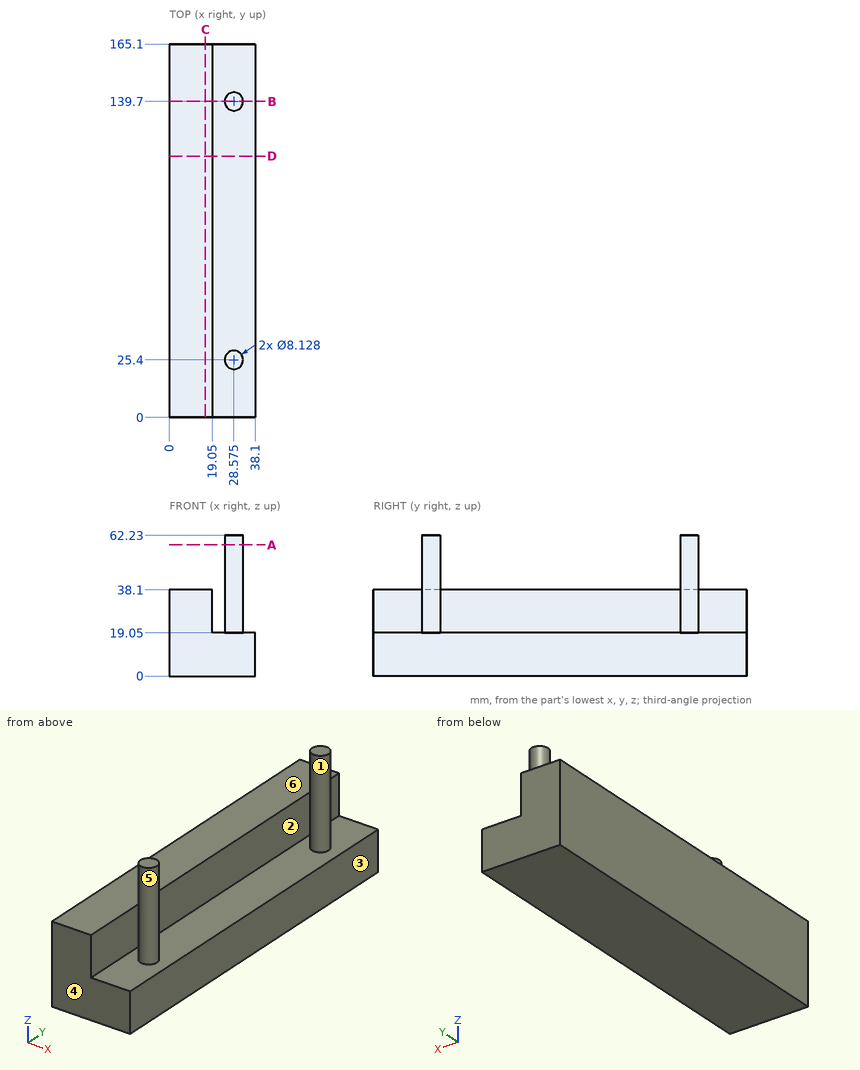
Answer from the drawing. Dimensions are ordinates in mm from the lowest x, y and z of the part. A direction names the side the tool comes from. Give positions to 0.01 mm unless a question says otherwise; leave off trailing zeros. Write each loop counter-clockwise with the first axis right and the second up, starting at its lowest first coordinate (ties: lowest second). Pieces come first, ordered by that corner, then holes. Notation, with made-up numbers: (-22, 64) - (1, 64) arc R19 cw to (1, 90) - close; hole circle Ø10 at (27, 40). An arc over 180 degrees is marked (long way). Answer in a Markdown table with one row per item. Add a question column.
Item 1: Find the intervals of material crossed by L1, parallel to Z at x = 36, y = 95; L2, parallel to Y at x = 28.5, z = 55.5; L3, parallel to Z at x = 18, y = 75, in increasing order.
Item 2: Section C-C, the plane x = 16 is taken. Write down the section's boundary in (y, z), and give its area (3 significant figures).
Item 3: Section A-A, the plane z = 58 is taken. Write down the section's boundary in (x, y) (3 decimals).
Item 4: A tool of negligible diameter and unlimited length cuts with its end or side. For the marked faces 1, 2 and 3, from which of +Z, -Z, +X, -X, +Y, -Y can it reach the whole face along a straight path? Write none if from no direction.
Item 5: Determine the mould class of the marked faces 4, 5 and 6 for opening direction Y: pulls with the +Y half, pulls with the -Y half, needs draft (parallel to the pull), parting line crosses it, or undercut.
Item 6: Section B-B, the plane y = 139.7 is taken. Write down the section's boundary in (x, z).
Item 7: Section D-D, the plane y = 115.5 is taken. Write down the section's boundary in (x, z).
Item 8: Flat-ended cylindrical pins translate along their axes: P1, Ø12, axis at y = 34.5, z = 30, coming from the +X side; P2, Ø15, axis at y = 68, z = 33, coming from the +X side; P3, Ø6, axis at y = 30.5, z = 35.5, coming from the -X side; P4, Ø6, axis at x = 9.5, z = 41.5, coming from the -Y side. Find the tip coordinate at first contact, or state that the pin passes through.
Recorded:
| question | item | result |
|---|---|---|
| 1 | L1 | z = 0 to 19.05 |
| 1 | L2 | y = 21.34 to 29.46, 135.64 to 143.76 |
| 1 | L3 | z = 0 to 38.1 |
| 2 | outline | (0, 0) - (165.1, 0) - (165.1, 38.1) - (0, 38.1) - close |
| 2 | area | 6,290 mm2 |
| 3 | outline | circle Ø8.128 at (28.575, 25.4); circle Ø8.128 at (28.575, 139.7) |
| 4 | face 1 | +Z |
| 4 | face 2 | +Z, +Y, -Y |
| 4 | face 3 | +Z, -Z, +X, +Y, -Y |
| 5 | face 4 | pulls with the -Y half |
| 5 | face 5 | undercut |
| 5 | face 6 | needs draft |
| 6 | outline | (0, 0) - (38.1, 0) - (38.1, 19.05) - (32.64, 19.05) - (32.64, 62.23) - (24.51, 62.23) - (24.51, 19.05) - (19.05, 19.05) - (19.05, 38.1) - (0, 38.1) - close |
| 7 | outline | (0, 0) - (38.1, 0) - (38.1, 19.05) - (19.05, 19.05) - (19.05, 38.1) - (0, 38.1) - close |
| 8 | P1 | stops at x = 31.2 |
| 8 | P2 | stops at x = 19.05 |
| 8 | P3 | stops at x = 0 |
| 8 | P4 | passes through |
